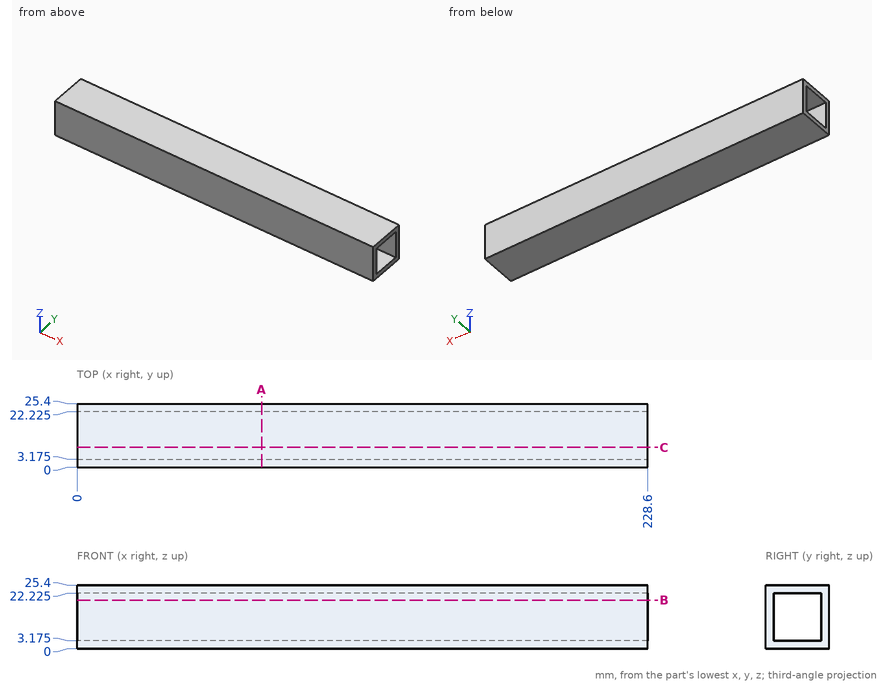
Can you work these out from the drawing? Everything is in mm from the part's minimum corner. Give positions to 0.01 mm unless a question says otherwise; leave off trailing zeros. Order: outer loops, then holes, each group sorted by start corner. A loop starts at its lowest first (then second) coordinate and runs counter-clockwise, first axis right, second up.
Item 1: If we section it at B-B, the plane z = 19.5: Write out the boundary of the cut face in (x, y) (3 decimals).
Item 2: I need wall thicknesses on line 1 (Y direction, x = 196, z = 11.25) (3 decimals). Which ranges of the line are inside material? Lowest first, please.
Item 3: I'm going to push a flat-ended pin straight in: pin 1 (15 mm diameter, centred on x = 115.5, y = 14.5, fed in from -Z). Where does the tip first touch, or does it pass through?
Item 4: If we section it at A-A, the plane x = 74: Write out the boundary of the cut face in (y, z) (3 decimals), plus the area to 3 significant figures.
Values:
1. outline: (0, 0) - (228.6, 0) - (228.6, 3.175) - (0, 3.175) - close; (0, 22.225) - (228.6, 22.225) - (228.6, 25.4) - (0, 25.4) - close
2. line 1: y = 0 to 3.175, 22.225 to 25.4
3. pin 1: stops at z = 0
4. outline: (0, 0) - (25.4, 0) - (25.4, 25.4) - (0, 25.4) - close; hole (3.175, 3.175) - (22.225, 3.175) - (22.225, 22.225) - (3.175, 22.225) - close
4. area: 282 mm2
